```python
from build123d import *

# Parameters (mm, degrees)
F1_DEPTH = 25.4
F2_DEPTH = 19.05
F4_DEPTH = 12.7
F6_DEPTH = 12.701
F8_DEPTH = 12.7


with BuildPart() as f1:
    # F0 (on Front) → F1 (new body)
    with BuildSketch(Plane.XZ):
        Polygon((-42.0901787708, 12.7), (-42.0200370051, 0), (-3.9200370051, 0), (-3.9200370051, 12.9108126882), align=None)
    extrude(amount=F1_DEPTH)

    # F2 (add): a face of the model
    f2_faces = [f1.faces().sort_by_distance(p)[0] for p in [
        (-23.005107888, -12.7, 12.8054063441),
    ]]
    extrude(f2_faces, amount=F2_DEPTH)

    # F3 (on face) → F4 (cut)
    with BuildSketch(Plane.XZ.offset(25.4)):
        Polygon((-42.0901787708, 12.7), (-3.9200370051, 12.9108126882), (-4.025248049, 31.9605221515), (-42.1953898147, 31.7497094633), align=None)
    extrude(amount=-F4_DEPTH, mode=Mode.SUBTRACT)

    # F5 (on face) → F6 (cut, through all)
    with BuildSketch(Plane.XZ.offset(12.7)):
        Polygon((-4.025248049, 31.9605221515), (-16.7250543579, 31.8903814555), (-3.9200370051, 12.9108126882), align=None)
    extrude(amount=-F6_DEPTH, mode=Mode.SUBTRACT)

    # F7 (on face) → F8 (cut)
    with BuildSketch(Plane(origin=(-0.0714234738, 0, 12.9320684794), x_dir=(0.9999847487, 0, 0.0055228894), z_dir=(-0.0055228894, 0, 0.9999847487))):
        Polygon((-3.8486722285, -12.7), (-16.5486722285, -25.4), (-3.8486722285, -25.4), align=None)
    extrude(amount=-F8_DEPTH, mode=Mode.SUBTRACT)


solid = f1.part
```
The model under review builds one solid part; all positions refer to its coordinate system, in mm. Give positions to 0.01 mm unless a question says otherwise; leave off trailing zeros. Write each loop counter-clockwise with the first axis right and the second up, starting at its lowest first coordinate (ties: lowest second). Pieces come first, ordered by that corner, then holes.
(1) Consider section D-D, the plane x = -7.5. Give the boundary of the cut face in (y, z), and give its area (3 significant figures).
(2) For P1, Ø12, axis at x = -36.5, y = -14, coming from the +Z side; P2, Ø1.5, axis at y = -3, z = 22, coming from the -X side; P3, Ø4, axis at y = -16.5, z = 14.5, coming from the +X side, all flat-tipped, find the tip position at first contact; note any pin that passes through.
(3) Consider section C-C, the plane y = -16.25. Give the boundary of the cut face in (x, z), and give its area (3 significant figures).
(4) Consider section B-B, the plane z = 5. Give the boundary of the cut face in (x, y), and give its area (3 significant figures).
(5) Consider section A-A, the plane x = -16. Give the boundary of the cut face in (y, z).
(6) To check wall thickness, follow L1, parallel to Z at x = -5.5, y = -21.5; L2, parallel to Y at x = -22, z = 20; L3, parallel to Z at x = -18, y = -21.25. State the ranges of each line that lie inside material, in increasing order.
Returned:
1. outline: (-25.4, 0) - (0, 0) - (0, 18.22) - (-12.7, 18.22) - (-12.7, 12.89) - (-16.28, 12.89) - (-16.35, 0.19) - (-25.4, 0.19) - close
1. area: 280 mm2
2. P1: stops at z = 31.81
2. P2: stops at x = -42.15
2. P3: stops at x = -6.52
3. outline: (-42.09, 12.7) - (-42.02, 0) - (-3.92, 0) - (-3.92, 0.21) - (-7.4, 0.19) - (-7.47, 12.89) - close
3. area: 444 mm2
4. outline: (-42.05, -25.4) - (-16.58, -25.4) - (-3.92, -12.74) - (-3.92, 0) - (-42.05, 0) - close
4. area: 888 mm2
5. outline: (-25.4, 0) - (0, 0) - (0, 30.82) - (-12.7, 30.82) - (-12.7, 12.84) - (-24.78, 12.84) - (-24.85, 0.14) - (-25.4, 0.14) - close
6. L1: z = 0 to 0.2
6. L2: y = -12.7 to 0
6. L3: z = 0 to 12.83
